Could you check a few things on this model? Use its own coordinates, in mm. A direction names the side the tool comes from. Give positions to 0.01 mm unless a question says otherwise; leave off trailing zeros. Order: outer loops, then holes, each group sorted by start corner. A loop starts at its lowest first (then second) coordinate and runs counter-clockwise, first axis right, second up. Notation, with made-up numbers: (18.5, 65.5) - (59.5, 65.5) arc R17 cw to (59.5, 89.5) - close; hole circle Ø7 at (-2, -38). An arc over 180 degrees is marked (long way). Put each result on its own line as item: value.
from build123d import *

# Parameters (mm, degrees)
F0_W     = 60
F0_H     = 120
F0_R     = 2.25
F1_DEPTH = 5
F2_W     = 5
F2_H     = 120
F3_DEPTH = 25
F4_W     = 21
F4_H     = 5.5
F5_DEPTH = 72
F6_R     = 1


with BuildPart() as f1:
    # F0 (on Front) → F1 (new body)
    with BuildSketch(Plane.XZ):
        Rectangle(F0_W, F0_H)
        with Locations((-20, -50)):
            Circle(F0_R, mode=Mode.SUBTRACT)
        with Locations((20, -50)):
            Circle(F0_R, mode=Mode.SUBTRACT)
        with Locations((-20, 50)):
            Circle(F0_R, mode=Mode.SUBTRACT)
        with Locations((20, 50)):
            Circle(F0_R, mode=Mode.SUBTRACT)
    extrude(amount=F1_DEPTH)

    # F2 (on face) → F3 (join)
    with BuildSketch(Plane(origin=(0, 0, 0), x_dir=(-1, 0, 0), z_dir=(0, 1, 0))):
        with Locations((-27.5, 0)):
            Rectangle(F2_W, F2_H)
        with Locations((27.5, 0)):
            Rectangle(F2_W, F2_H)
    extrude(amount=F3_DEPTH)

    # F4 (on face) → F5 (cut)
    with BuildSketch(Plane(origin=(-30, 0, 0), x_dir=(0, -1, 0), z_dir=(-1, 0, 0))):
        with Locations((-14.5, 32.75)):
            Rectangle(F4_W, F4_H)
        with BuildLine():
            ThreePointArc((-4, 30), (-1.25, 32.75), (-4, 35.5))
            Line((-4, 35.5), (-4, 30))
        make_face()
        with Locations((-14.5, -27.25)):
            Rectangle(F4_W, F4_H)
        with BuildLine():
            ThreePointArc((-4, -30), (-1.25, -27.25), (-4, -24.5))
            Line((-4, -24.5), (-4, -30))
        make_face()
    extrude(amount=-F5_DEPTH, mode=Mode.SUBTRACT)

    # F6
    f6_edges = [f1.edges().sort_by_distance(p)[0] for p in [
        (-27.5, 25, 35.5),
        (27.5, 25, 30),
        (27.5, 25, 35.5),
        (-27.5, 25, 30),
        (27.5, 25, -24.5),
        (-27.5, 25, -24.5),
        (-27.5, 25, -30),
        (27.5, 25, -30),
    ]]
    fillet(f6_edges, radius=F6_R)


solid = f1.part
1) Suppose I cut it at D-D, the plane z = -45.5. List the corners of the cut face in (x, y) for me.
Filled in:
outline: (-30, -5) - (30, -5) - (30, 25) - (25, 25) - (25, 0) - (-25, 0) - (-25, 25) - (-30, 25) - close
2) Suppose I cut it at A-A, the plane x = 20. List the corners of the cut face in (y, z) for me.
Filled in:
outline: (-5, -60) - (0, -60) - (0, -52.25) - (-5, -52.25) - close; (-5, -47.75) - (0, -47.75) - (0, 47.75) - (-5, 47.75) - close; (-5, 52.25) - (0, 52.25) - (0, 60) - (-5, 60) - close
3) I'm going to push flat-ended pins straight in: pin 1 (6 mm diameter, centred on x = 2, z = -48, fed in from +Y); pin 2 (3 mm diameter, centred on x = -23, y = 10.5, fed in from +Z). Where does each tip first touch, or does it pass through?
Filled in:
pin 1: stops at y = 0
pin 2: passes through
4) If I drill on line 1 (Z direction, x = -20, y = -3.2); line 2 (Z direction, x = -25.5, y = 5.5); line 3 (X direction, y = 15, z = -51.5), over which ranges is the centre line in solid material (lowest first)? Write a range as [from, to].
Filled in:
line 1: z = [-60, -52.25], [-47.75, 47.75], [52.25, 60]
line 2: z = [-60, -30], [-24.5, 30], [35.5, 60]
line 3: x = [-30, -25], [25, 30]
5) Suppose I cut it at B-B, the plane y = 10. List the corners of the cut face in (x, z) for me.
Filled in:
outline: (-30, -60) - (-25, -60) - (-25, -30) - (-30, -30) - close; (-30, -24.5) - (-25, -24.5) - (-25, 30) - (-30, 30) - close; (-30, 35.5) - (-25, 35.5) - (-25, 60) - (-30, 60) - close; (25, -60) - (30, -60) - (30, -30) - (25, -30) - close; (25, -24.5) - (30, -24.5) - (30, 30) - (25, 30) - close; (25, 35.5) - (30, 35.5) - (30, 60) - (25, 60) - close
6) Which directions (+Z, -Z, +X, -X, +Y, -Y) give clear straight access to the entire face, cutting with the end or side of a thin tool? Please do faces 1 (the flat face through (27, 14, 30)), 2 (the flat face through (-27, 25, 48)), 3 (the flat face through (0, 0, 1)).
Filled in:
face 1: +X, -X, +Y
face 2: +Z, -Z, +X, -X, +Y
face 3: +Z, -Z, +Y
7) Suppose I cut it at C-C, the plane z = -27.25. List the corners of the cut face in (x, y) for me.
Filled in:
outline: (-30, -5) - (30, -5) - (30, 1.25) - (25, 1.25) - (25, 0) - (-25, 0) - (-25, 1.25) - (-30, 1.25) - close
8) We'd pull the mould along Z, two halves only. Please class faces 4 (the flat face through (-28, 14, -30)), 5 (the flat face through (0.4, -0.2, 60)), 6 (the flat face through (0.4, -0.2, -60)), 7 (the flat face through (28, 25, 48)): pulls with the +Z half, pulls with the -Z half, needs draft (parallel to the pull), parting line crosses it, or undercut.
Filled in:
face 4: undercut
face 5: pulls with the +Z half
face 6: pulls with the -Z half
face 7: needs draft
